Here's how the part is built. I have some questions about the finished solid (model axes, mm). A direction names the side the tool comes from. Coordinates: 2 decimals unless noted, no trailing zeros. Write each loop counter-clockwise with the first axis right and the second up, starting at its lowest first coordinate (ties: lowest second). Pieces come first, ordered by that corner, then holes. Notation, with made-up numbers: M -18.75,-17.75 L 38.25,-17.75 A20 cw 38.25,-5.75 Z; hole C 1,7.25 d5. An arc over 180 degrees is marked long. Use one line per item in the form item = value. Start each with the question number.
1. Please list where these lines run through material, in increasing order: line 1 along Z through (x, y) = (5.5, 0); line 2 along X through (y, z) = (0.25, -3.5); line 3 along Y through (x, z) = (41, -0.25). Write a range as [from, to].
2. I want a section at D-D, the plane x = 18. List the corners of the cut face in (y, z) for me (1 decimal).
3. I want a section at A-A, the plane y = 0. List the corners of the cut face in (x, z) for me.
4. I want a section at B-B, the plane x = 48.5. List the corners of the cut face in (y, z) for me, plus the area to 3 significant figures.
5. On a 3-axis mill with a long thin cutter (end or side, diameter ignored), from which of +Z, -Z, +X, -X, +Y, -Y can I reach the whole of each face in a straight line? I mean faces 1 (the face through (50.399, -3.2, -2.454)), 2 (the face through (39.878, 0, -2)). Say none if no direction works.
6. I'm going to push flat-ended pins straight in: pin 1 Ø4 at (x, z) = (34, 2.5) entering from +Y; pin 2 Ø1.5 at (x, z) = (35, 3) entering from +Y. Where does each tip first touch, or does it pass through?
7. I want a section at C-C, the plane z = 2.5. List the corners of the cut face in (x, y) for me, plus the area to 3 significant figures.
Autodesk Inventor part; units mm, degrees
ref_plane "dia1_XY" through (0, 1.5875, 0) normal (1, 0, 0) x (0, 0, -1)
ref_plane "dia1_YZ" through (0, 1.5875, 0) normal (0, 0, -1) x (0, 1, 0)
ref_plane "dia1_ZX" through (0, 1.5875, 0) normal (0, 1, 0) x (1, 0, 0)
sketch "Sketch_1" plane through (0, 0, 0) normal (0, 0, 1) x (1, 0, 0)
  line L0 (60.6298, 0) -> (0, 0)
  line L1 (0, 0) -> (0, 1.5875)
  line L2 (0, 1.5875) -> (39.878, 1.5875)
  line L3 (39.878, 1.5875) -> (39.878, 4.0323)
  line L4 (39.878, 4.0323) -> (60.6298, 4.0323)
  line L5 (60.6298, 4.0323) -> (60.6298, 0)
  line L6 (60.6298, 0) -> (0, 0)
revolve "Revolution1" add sketch "Sketch_1" angle 360 about axis through (60.6298, 0, 0) along (1, 0, 0)
sketch "Sketch_2" plane through (0, 0, 0) normal (0, 0, 1) x (1, 0, 0)
  line L0 (0, 0) -> (-9.652, 0)
  line L1 (-9.652, 0) -> (-9.652, 1.209)
  line L2 (-9.652, 1.209) -> (-9.2735, 1.5875)
  line L3 (-9.2735, 1.5875) -> (0, 1.5875)
  line L4 (0, 1.5875) -> (0, 0)
  line L5 (0, 0) -> (-9.652, 0)
revolve "Revolution2" add sketch "Sketch_2" angle 360 about axis through (0, 0, 0) along (1, 0, 0)
sketch "Sketch_30" plane through (0, 0, 0) normal (0, 0, 1) x (1, 0, 0)
  line L0 (0, 0) -> (-0.254, 0)
  line L1 (-0.254, 1.3335) -> (0, 1.3335)
  line L2 (0, 1.3335) -> (0, 1.8415)
  line L3 (0, 1.8415) -> (-0.254, 1.8415)
  line L4 (-0.254, 1.8415) -> (-0.254, 1.3335)
revolve "Revolution3" cut sketch "Sketch_30" angle 360 about axis through (0, 0, 0) along (1, 0, 0)
ref_plane "dia1_XY" through (0, 1.5875, 0) normal (1, 0, 0) x (0, 0, -1)
ref_plane "dia1_YZ" through (0, 1.5875, 0) normal (0, 0, -1) x (0, 1, 0)
ref_plane "dia1_ZX" through (0, 1.5875, 0) normal (0, 1, 0) x (1, 0, 0)
ref_plane "dia12_XY" through (0, 0, 7.6835) normal (1, 0, 0) x (0, 0, -1)
ref_plane "dia12_YZ" through (0, 0, 7.6835) normal (0, 0, -1) x (0, 1, 0)
ref_plane "dia12_ZX" through (0, 0, 7.6835) normal (0, 1, 0) x (1, 0, 0)
ref_plane "dia1r_XY" through (0, 0, 4.5593) normal (1, 0, 0) x (0, 0, -1)
ref_plane "dia1r_YZ" through (0, 0, 4.5593) normal (0, 0, -1) x (0, 1, 0)
ref_plane "dia1r_ZX" through (0, 0, 4.5593) normal (0, 1, 0) x (1, 0, 0)
ref_plane "dia2_XY" through (0, -1.5875, 0) normal (1, 0, 0) x (0, 0, -1)
ref_plane "dia2_YZ" through (0, -1.5875, 0) normal (0, 0, -1) x (0, 1, 0)
ref_plane "dia2_ZX" through (0, -1.5875, 0) normal (0, 1, 0) x (1, 0, 0)
ref_plane "dia22_XY" through (0, 0, -7.6835) normal (1, 0, 0) x (0, 0, -1)
ref_plane "dia22_YZ" through (0, 0, -7.6835) normal (0, 0, -1) x (0, 1, 0)
ref_plane "dia22_ZX" through (0, 0, -7.6835) normal (0, 1, 0) x (1, 0, 0)
ref_plane "dia2r_XY" through (0, 0, -4.5593) normal (1, 0, 0) x (0, 0, -1)
ref_plane "dia2r_YZ" through (0, 0, -4.5593) normal (0, 0, -1) x (0, 1, 0)
ref_plane "dia2r_ZX" through (0, 0, -4.5593) normal (0, 1, 0) x (1, 0, 0)
ref_plane "rl1_XY" through (-9.652, 0, 0) normal (1, 0, 0) x (0, 0, -1)
ref_plane "rl1_YZ" through (-9.652, 0, 0) normal (0, 0, -1) x (0, 1, 0)
ref_plane "rl1_ZX" through (-9.652, 0, 0) normal (0, 1, 0) x (1, 0, 0)
ref_plane "rl2_XY" through (0, 0, 0) normal (1, 0, 0) x (0, 0, -1)
ref_plane "rl2_YZ" through (0, 0, 0) normal (0, 0, -1) x (0, 1, 0)
ref_plane "rl2_ZX" through (0, 0, 0) normal (0, 1, 0) x (1, 0, 0)
ref_plane "rod_cp_XY" through (0, 0, 0) normal (1, 0, 0) x (0, 0, -1)
ref_plane "rod_cp_YZ" through (0, 0, 0) normal (0, 0, -1) x (0, 1, 0)
ref_plane "rod_cp_ZX" through (0, 0, 0) normal (0, 1, 0) x (1, 0, 0)
ref_plane "stroke1_XY" through (0, 0, 0) normal (1, 0, 0) x (0, 0, -1)
ref_plane "stroke1_YZ" through (0, 0, 0) normal (0, 0, -1) x (0, 1, 0)
ref_plane "stroke1_ZX" through (0, 0, 0) normal (0, 1, 0) x (1, 0, 0)
ref_plane "thd1_XY" through (-9.652, 1.5875, 0) normal (1, 0, 0) x (0, 0, -1)
ref_plane "thd1_YZ" through (-9.652, 1.5875, 0) normal (0, 0, -1) x (0, 1, 0)
ref_plane "thd1_ZX" through (-9.652, 1.5875, 0) normal (0, 1, 0) x (1, 0, 0)
ref_plane "thd2_XY" through (-9.652, -1.5875, 0) normal (1, 0, 0) x (0, 0, -1)
ref_plane "thd2_YZ" through (-9.652, -1.5875, 0) normal (0, 0, -1) x (0, 1, 0)
ref_plane "thd2_ZX" through (-9.652, -1.5875, 0) normal (0, 1, 0) x (1, 0, 0)
ref_plane "to_rod_clevis_XY" through (-9.652, 0, 0) normal (1, 0, 0) x (0, 0, -1)
ref_plane "to_rod_clevis_YZ" through (-9.652, 0, 0) normal (0, 0, -1) x (0, 1, 0)
ref_plane "to_rod_clevis_ZX" through (-9.652, 0, 0) normal (0, 1, 0) x (1, 0, 0)
properties part number "0070.725-R0000_rod"
Answer list:
q1.line_1 = [-1.59, 1.59]
q1.line_2 = [39.88, 60.63]
q1.line_3 = [-4.02, 4.02]
q2.outline = C 0,0 d3.2
q3.outline = M -9.65,-1.21 L -9.27,-1.59 L -0.25,-1.59 L -0.25,-1.33 L 0,-1.33 L 0,-1.59 L 39.88,-1.59 L 39.88,-4.03 L 60.63,-4.03 L 60.63,4.03 L 39.88,4.03 L 39.88,1.59 L 0,1.59 L 0,1.33 L -0.25,1.33 L -0.25,1.59 L -9.27,1.59 L -9.65,1.21 Z
q4.outline = C 0,0 d8.06
q4.area = 51.1 mm²
q5.face_1 = +X, -X
q5.face_2 = -X
q6.pin_1 = 1.51
q6.pin_2 = through
q7.outline = M 39.88,-3.16 L 60.63,-3.16 L 60.63,3.16 L 39.88,3.16 Z
q7.area = 131 mm²
